Source: CAD feature listing. Evaluate the final solid. Frame: model axes, mm. Face numbers are marked on the shaded views. A direction names the side the tool comes from. Round coordinates to 2 decimals unless told otherwise and drop trailing zeros. Loops run counter-clockwise (first coordinate to the right, second up) from the corner with the lowest first, then second, coordinate; pieces in that order, holes last. Notation, with made-up numbers: M 86.5,76.25 L 99.5,76.25 A8 ccw 99.5,81.25 Z; hole C 82,51.5 d8. An arc over 180 degrees is marked long. Answer as a JSON object with one key per item and string values.
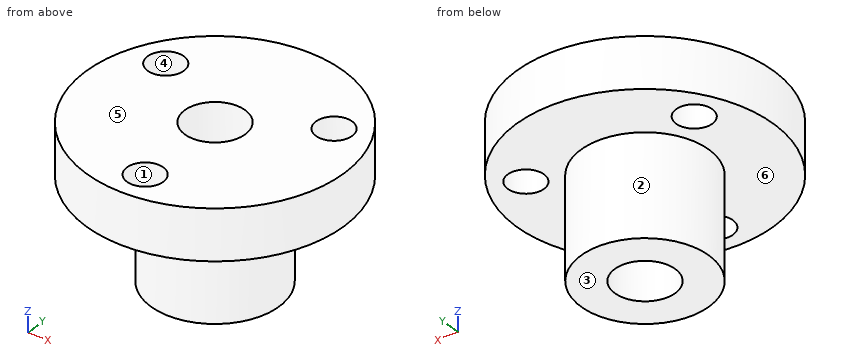
Autodesk Inventor part; units mm, degrees
ref_plane "YZ Plane" through (0, 0, 0) normal (1, 0, 0) x (0, 1, 0)
ref_plane "XZ Plane" through (0, 0, 0) normal (0, 1, 0) x (-1, 0, 0)
ref_plane "XY Plane" through (0, 0, 0) normal (0, 0, 1) x (1, 0, 0)
sketch "Sketch1" plane through (0, 0, 0) normal (0, 0, 1) x (1, 0, 0)
  line L0 (-17.85, 0) -> (17.85, 0) construction
  line L1 (0, -17.85) -> (0, 17.85) construction
  circle A0 centre (0, 0) radius 12.75
  dimension "d0" = 25.5
extrude "Extrusion1" add sketch "Sketch1" along normal blind 5
sketch "Sketch2" plane through (0, 0, 0) normal (0, 0, -1) x (-1, 0, 0)
  circle A0 centre (0, 0) radius 6.35
  dimension "d3" = 12.7
extrude "Extrusion2" add sketch "Sketch2" along normal blind 10
sketch "Sketch3" plane through (0, 0, -10) normal (0, 0, -1) x (-1, 0, 0)
  circle A0 centre (0, 0) radius 3
  dimension "d6" = 6
extrude "Extrusion3" cut sketch "Sketch3" against normal through all
sketch "Sketch5" plane through (0, 0, 5) normal (0, 0, 1) x (1, 0, 0)
  circle A0 centre (0, 0) radius 9.525 construction
  circle A1 centre (0, -9.525) radius 1.8
  line L0 (-17.85, 0) -> (17.85, 0) construction
  line L1 (0, -17.85) -> (0, 17.85) construction
  circle A2 centre (8.2489, 4.7625) radius 1.8
  circle A3 centre (-8.2489, 4.7625) radius 1.8
  dimension "d13" = 19.05
  dimension "d14" = 3.6
  dimension "d19" = 360
extrude "Extrusion5" cut sketch "Sketch5" against normal through all
properties part number "Nakretka_prowadnica_tloka"
Item 1: Contact query for flat-ended pins moving along their axis: pin 1 Ø6 at (x, y) = (8.25, 4.76) entering from -Z; pin 2 Ø2 at (y, z) = (-9, -6) entering from -X (3 decimals); pin 3 Ø5 at (x, z) = (5, -4.5) entering from +Y; pin 4 Ø5 at (y, z) = (3, -5.5) entering from -X. Output: stop coordinate, or through.
Answer sheet:
{"pin 1": "stops at z = 0", "pin 2": "passes through", "pin 3": "stops at y = 5.84", "pin 4": "stops at x = -6.33"}
Item 2: Section C-C on y = -10.5. Return the cut outline in (x, z), then the cut area to 3 significant figures.
Answer sheet:
{"outline": "M -7.23,0 L -1.51,0 L -1.51,5 L -7.23,5 Z; M 1.51,0 L 7.23,0 L 7.23,5 L 1.51,5 Z", "area": "57.2 mm²"}
Item 3: Section B-B on x = 0. Return the cut outline in (y, z) (3 decimals).
Answer sheet:
{"outline": "M -12.75,0 L -11.325,0 L -11.325,5 L -12.75,5 Z; M -7.725,0 L -6.35,0 L -6.35,-10 L -3,-10 L -3,5 L -7.725,5 Z; M 3,-10 L 6.35,-10 L 6.35,0 L 12.75,0 L 12.75,5 L 3,5 Z"}
Item 4: Line query: probe 1 along Y at (x, z) = (0, 1.5) (3 decimals); probe 2 along Y at (x, z) = (0, -3.75); probe 3 along Y at (x, z) = (2.5, 0.25). Output: solid intervals per line, ascending. Write a range as from..to.
Answer sheet:
{"probe 1": "y = -12.75..-11.325, -7.725..-3, 3..12.75", "probe 2": "y = -6.35..-3, 3..6.35", "probe 3": "y = -12.5..-1.66, 1.66..12.5"}
Item 5: Section D-D on z = -5.75. Return the cut outline in (x, y), then the cut area to 3 significant figures.
Answer sheet:
{"outline": "C 0,0 d12.7; hole C 0,0 d6", "area": "98.4 mm²"}
Item 6: Access query for the marked faces 5 and 6. Directions: +Z, -Z, +X, -X, +Y, -Y. A direction counts if a zero-diameter tool reaches every point of the face in a straight line with its end or side. Return the directions, or none.
Answer sheet:
{"face 5": "+Z, +X, -X, +Y, -Y", "face 6": "-Z"}
Item 7: Section A-A on y = 0. Return the cut outline in (x, z), then the cut area to 4 significant figures.
Answer sheet:
{"outline": "M -12.75,0 L -6.35,0 L -6.35,-10 L -3,-10 L -3,5 L -12.75,5 Z; M 3,-10 L 6.35,-10 L 6.35,0 L 12.75,0 L 12.75,5 L 3,5 Z", "area": "164.5 mm²"}
Item 8: Pull-direction query (X, two-part tool) for the marked faces 1, 2, 3 and 4; classes: pulls with the +X half, pulls with the -X half, needs draft (parallel to the pull), parting line crosses it, or undercut.
Answer sheet:
{"face 1": "undercut", "face 2": "parting line crosses it", "face 3": "needs draft", "face 4": "undercut"}
